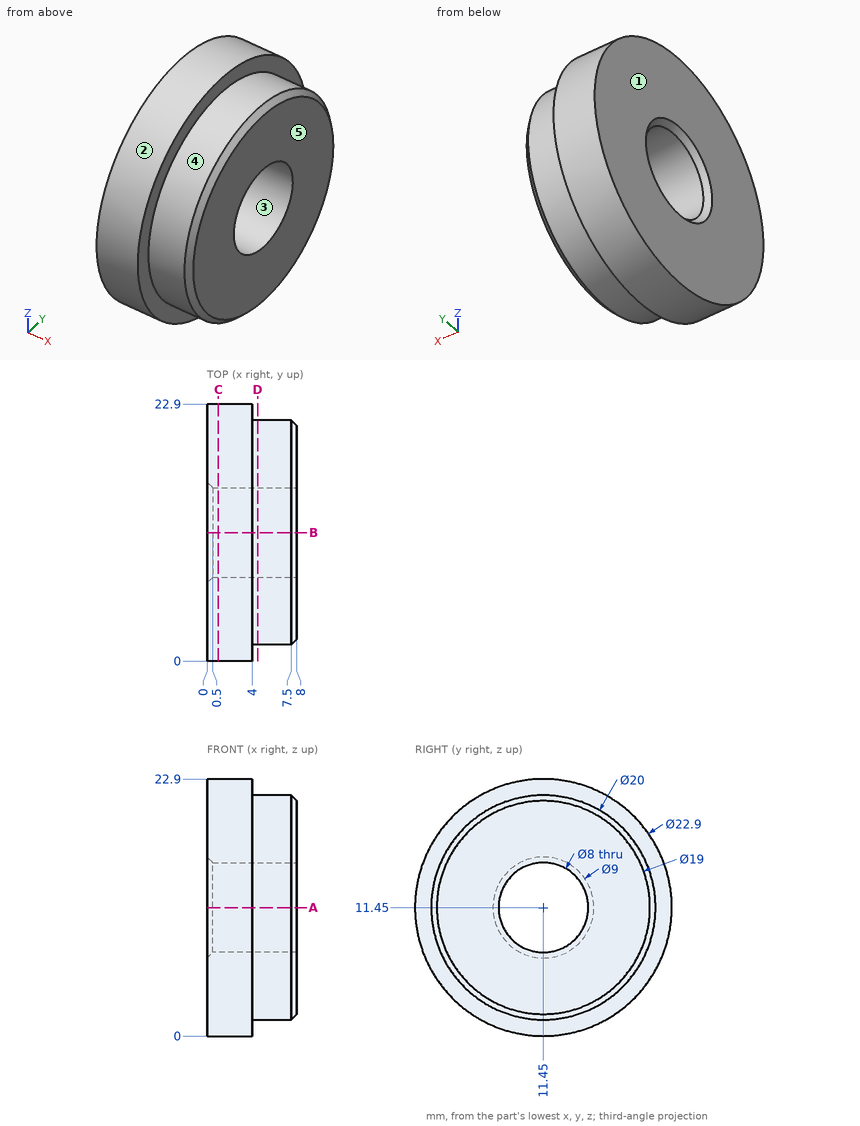
For this review, use the dimensioned drawing (mm, ordinates from the lowest corner) and the shaded views. A direction names the side the tool comes from. Give positions to 0.01 mm unless a question says otherwise; leave off trailing zeros. Order: outer loops, then holes, each group sorted by start corner. A loop starts at its lowest first (then second) coordinate and runs counter-clockwise, first axis right, second up. Notation, with made-up numbers: (72, -34) - (131, -34) arc R12 ccw to (131, -15) - close; hole circle Ø6 at (59, 67). An arc over 180 degrees is marked (long way). Use CSV: the item, a comma, the result in double quotes. Start each with the question number.
Q1. We need section D-D, the plane x = 4.5. Write out the cut boundary in (y, z).
Q2. We need section C-C, the plane x = 1. Write out the cut boundary in (y, z), and give its area (3 significant figures).
Q3. Tool access review of the marked faces 4 and 5: name each direction out of +Z, -Z, +X, -X, +Y, -Y from which nothing blocks a thin tool from reaching the whole face with its end or side.
Q4. The part is to be moulded in two halves that separate along Y. For the marked faces 1, 2 and 3, say which applies: +Y half, -Y half, draft (parallel to the pull), parting line (faces both ways), or undercut.
Q5. To check wall thickness, follow line 1 along Y through (x, z) = (3.5, 11.45); line 2 along Y through (x, z) = (4.25, 11.45); line 3 along X through (y, z) = (18.75, 4.25). State the ranges of each line that lie inside material, in increasing order. Write a range as [from, to].
Q6. Clearance check with flat-ended pins moving along their axes: pin 1 Ø3 at (x, y) = (4.5, 7.5) entering from -Z; pin 2 Ø1 at (x, y) = (3, 2.5) entering from +Z. State where each tip first meets the part, or that it passes through.
Q7. We need section A-A, the plane z = 11.45. Write out the cut boundary in (x, y), and give its area (3 significant figures).
Outcome:
1,outline,"circle Ø20 at (11.45, 11.45); hole circle Ø8 at (11.45, 11.45)"
2,outline,"circle Ø22.9 at (11.45, 11.45); hole circle Ø8 at (11.45, 11.45)"
2,area,"362 mm^2"
3,face 4,"+X"
3,face 5,"+Z, -Z, +X, +Y, -Y"
4,face 1,"draft"
4,face 2,"parting line"
4,face 3,"undercut"
5,line 1,"y = [0, 7.45], [15.45, 22.9]"
5,line 2,"y = [1.45, 7.45], [15.45, 21.45]"
5,line 3,"x = [0, 4]"
6,pin 1,"stops at z = 0.28"
6,pin 2,"stops at z = 19.18"
7,outline,"(0, 0) - (4, 0) - (4, 1.45) - (7.5, 1.45) - (8, 1.95) - (8, 7.45) - (0.5, 7.45) - (0, 6.95) - close; (0, 15.95) - (0.5, 15.45) - (8, 15.45) - (8, 20.95) - (7.5, 21.45) - (4, 21.45) - (4, 22.9) - (0, 22.9) - close"
7,area,"107 mm^2"
